Source: CAD feature listing. Evaluate the final solid. Frame: model axes, mm. A direction names the side the tool comes from. Give positions to 0.01 mm unless a question says otherwise; leave off trailing zeros. Write each loop counter-clockwise with the first axis right and the second up, starting at its lowest first coordinate (ties: lowest second). Pieces come first, ordered by that corner, then holes. Notation, with made-up numbers: (53.25, -4) -> (83.25, -4) arc R32 ccw to (83.25, 24) -> close; hole circle Ø8 at (-35, 6). An arc over 180 degrees is marked (long way). Answer as a JSON object with one key per item and string values. Group by question number.
Item 1: Section query A-A on z = -35. Return the cut outline in (x, y), plus the area to 3 significant figures.
Item 2: First-contact query: pin 1 Ø7.5 at (x, y) = (35, 4) entering from -Z; pin 2 Ø9 at (x, y) = (20.5, 14) entering from -Z; pin 3 Ø3 at (x, z) = (9, -17.5) entering from +Y. Flat tips, straight axial feed; report the tip coordinate or a pass-through.
Item 3: Section query C-C on y = 23. Return the cut outline in (x, z).
Item 4: Ray query, probe 1 along X at (y, z) = (16.25, -20.5); probe 2 along Z at (x, y) = (19.5, 9.5); probe 3 along Y at (x, z) = (2.25, -35). Return the intervals inside material, ascending. Write a range as from..to.
Item 5: Pull-direction query (X, two-part tool) for faces 4 (the face through (21.2, 3.2, -24.7)), 5 (the face through (37, 4, -31)), 6 (the face through (8.02, 7.15, -35.93)); classes: pulls with the +X half, pulls with the -X half, needs draft (parallel to the pull), parting line crosses it, or undercut.
Item 6: Access query for faces 1 (the face through (21, 0, -2)), 2 (the face through (4.727, 7.082, -2.465)), 3 (the face through (21, 10, -15)). Directions: +Z, -Z, +X, -X, +Y, -Y. A direction counts if a zero-diameter tool reaches every point of the face in a straight line with its end or side. Return the directions, or none.
Item 7: Section query D-D on z = -9. Return the cut outline in (x, y), plus the area to 3 significant figures.
Item 8: Section query B-B on x = 33.5. Return the cut outline in (y, z).
Autodesk Inventor part; units mm, degrees
ref_plane "YZ Plane" through (0, 0, 0) normal (1, 0, 0) x (0, 1, 0)
ref_plane "XZ Plane" through (0, 0, 0) normal (0, 1, 0) x (-1, 0, 0)
ref_plane "XY Plane" through (0, 0, 0) normal (0, 0, 1) x (1, 0, 0)
sketch "Sketch1" plane through (0, 0, 0) normal (1, 0, 0) x (0, 1, 0)
  line L0 (0, 0) -> (0, -5)
  line L1 (0, -5) -> (20, -5)
  line L2 (20, -5) -> (20, -15)
  line L3 (20, -15) -> (0, -15)
  line L4 (0, -15) -> (0, -39.4721)
  line L5 (25, 0) -> (25, -24)
  line L6 (25, -24) -> (7, -24)
  line L7 (7, -24) -> (7, -29.8038)
  line L8 (25, 0) -> (0, 0)
  circle A0 centre (4, -35) radius 3
  arc A1 (0, -39.4721) -> (7, -29.8038) centre (4, -35) ccw
  dimension "d0" = 5
  dimension "d1" = 20
  dimension "d2" = 10
  dimension "d5" = 5
  dimension "d6" = 7
  dimension "d7" = 6
  dimension "d8" = 20
  dimension "d9" = 4
  dimension "d10" = 6
  dimension "d45" = 9
extrude "Extrusion1" add sketch "Sketch1" along normal blind 42
fillet "Fillet1" radius 5 1 edges at (21, 25, 0)
sketch "Sketch2" plane through (0, 7, -24) normal (0, 1, 0) x (1, 0, 0)
  arc A0 (10.8664, 7) -> (31.1336, 7) centre (21, 12) ccw
  line L0 (0, 0) -> (42, 0)
  line L1 (10.8664, 7) -> (3.3664, 19.9904)
  line L2 (10.8664, 7) -> (25.8664, 7) construction
  line L3 (31.1336, 7) -> (38.6336, 19.9904)
  line L4 (31.1336, 7) -> (46.1336, 7) construction
  line L5 (38.6336, 19.9904) -> (3.3664, 19.9904)
  line L6 (0, 0) -> (42, 0)
  point P0 (0, -24)
  point P1 (21, 0)
  dimension "d14" = 11.3
  dimension "d15" = 12
  dimension "d16" = 7
  dimension "d17" = 15
  dimension "d18" = 120
  dimension "d19" = 15
  dimension "d20" = 60
extrude "Extrusion2" cut sketch "Sketch2" along normal through all both and the other way through all
sketch "Sketch3" plane through (42, 0, 0) normal (1, 0, 0) x (0, 0, -1)
  line L0 (29, 7) -> (31, 7)
  line L1 (31, 7) -> (31, 0)
  line L2 (31, 0) -> (43, 0)
  line L3 (43, 0) -> (43, 12)
  line L4 (43, 12) -> (29, 12)
  line L5 (29, 12) -> (29, 7)
  line L6 (15, 20) -> (15, 0)
  point P0 (0, 0)
  dimension "d23" = 7
  dimension "d24" = 16
  dimension "d25" = 2
  dimension "d26" = 12
  dimension "d27" = 14
extrude "Extrusion3" cut sketch "Sketch3" against normal up to surface
sketch "Sketch4" plane through (0, 25, -24) normal (0, 1, 0) x (1, 0, 0)
  circle A0 centre (5.5, -3.5) radius 1.6
  circle A1 centre (36.5, -3.5) radius 1.6
  line L0 (0, 0) -> (0, -19)
  line L1 (42, 0) -> (42, -19)
  line L2 (0, 0) -> (42, 0)
  point P0 (0, -24)
  dimension "d30" = 3.2
  dimension "d31" = 5.5
  dimension "d32" = 5.5
  dimension "d33" = 3.5
  dimension "d34" = 3.5
extrude "Extrusion4" cut sketch "Sketch4" against normal through all
sketch "Sketch5" plane through (0, 0, 0) normal (0, 0, 1) x (1, 0, 0)
  circle A0 centre (5, 5) radius 2.1
  circle A1 centre (37, 5) radius 2.1
  line L0 (0, 0) -> (42, 0)
  line L1 (0, 20) -> (0, 0)
  line L2 (42, 20) -> (42, 0)
  dimension "d37" = 4.2
  dimension "d38" = 5
  dimension "d39" = 5
  dimension "d40" = 5
extrude "Extrusion5" cut sketch "Sketch5" against normal up to next
sketch "Sketch6" plane through (0, 25, -24) normal (0, 1, 0) x (1, 0, 0)
  spline S0 degree 2 poles (24.4322, -4.6341) (24.4322, -4.7612) (24.4049, -5.0608) knots 0 0 0 1 1 1
  spline S1 degree 2 poles (24.4049, -5.0608) (24.3777, -5.3696) (24.3777, -5.5149) knots 0 0 0 1 1 1
  spline S2 degree 2 poles (24.3777, -5.5149) (24.3777, -6.9405) (24.8045, -8.2754) knots 0 0 0 1 1 1
  spline S3 degree 2 poles (24.8045, -8.2754) (24.977, -8.8293) (24.977, -9.0654) knots 0 0 0 1 1 1
  spline S4 degree 2 poles (24.977, -9.0654) (24.977, -9.3832) (24.4776, -9.7374) (24.2506, -9.7374) knots 0 0 0 1 2 2 2
  spline S5 degree 2 poles (24.2506, -9.7374) (24.1507, -9.7374) (23.7693, -9.6465) knots 0 0 0 1 1 1
  spline S6 degree 2 poles (23.7693, -9.6465) (23.288, -9.5285) (22.6796, -9.4559) knots 0 0 0 1 1 1
  line L0 (22.6796, -9.4559) -> (18.3573, -8.9837)
  spline S7 degree 2 poles (18.3573, -8.9837) (17.7398, -8.9292) (17.3766, -8.8384) (17.086, -8.4752) (17.086, -8.1573) knots 0 0 0 1 2 3 3 3
  spline S8 degree 2 poles (17.086, -8.1573) (17.086, -7.9122) (17.4583, -7.5308) (17.6762, -7.5308) knots 0 0 0 1 2 2 2
  spline S9 degree 2 poles (17.6762, -7.5308) (17.876, -7.5308) (18.3845, -7.6307) knots 0 0 0 1 1 1
  spline S10 degree 2 poles (18.3845, -7.6307) (19.12, -7.7669) (23.2608, -8.2572) (23.3879, -8.2572) knots 0 0 0 1 2 2 2
  spline S11 degree 2 poles (23.3879, -8.2572) (23.5332, -8.2572) (23.5332, -8.2027) knots 0 0 0 1 1 1
  spline S12 degree 2 poles (23.5332, -8.2027) (23.5332, -8.003) (23.397, -7.1131) knots 0 0 0 1 1 1
  spline S13 degree 2 poles (23.397, -7.1131) (23.3243, -6.6954) (23.3062, -6.2686) knots 0 0 0 1 1 1
  spline S14 degree 2 poles (23.3062, -6.2686) (23.2517, -5.0518) (23.1246, -4.5614) knots 0 0 0 1 1 1
  spline S15 degree 2 poles (23.1246, -4.5614) (23.0882, -4.407) (23.0882, -4.3344) knots 0 0 0 1 1 1
  spline S16 degree 2 poles (23.0882, -4.3344) (23.0882, -4.0438) (23.4333, -3.7169) (23.6694, -3.7169) knots 0 0 0 1 2 2 2
  spline S17 degree 2 poles (23.6694, -3.7169) (24.0145, -3.7169) (24.4322, -4.2799) (24.4322, -4.6341) knots 0 0 0 1 2 2 2
  point P0 (0, -24)
  point P1 (17.086, -10.4002)
extrude "Extrusion6" add sketch "Sketch6" along normal blind 0.6
equation "\"d32\" = d31"
equation "\"d40\" = d39"
properties material "ABS Plastic"
Worked answers:
{
 "1": {"outline": "(0, 0) -> (8.56, 0) -> (8.56, 1) -> (0, 1) -> close; (0, 7) -> (8.56, 7) -> (8.56, 10) -> (0, 10) -> close", "area": "34.2 mm^2"},
 "2": {"pin 1": "z = -31", "pin 2": "z = -24", "pin 3": "y = 25"},
 "3": {"outline": "(0, -24) -> (42, -24) -> (42, -1) -> (0, -1) -> close; hole circle Ø3.2 at (5.5, -20.5); hole circle Ø3.2 at (36.5, -20.5)"},
 "4": {"probe 1": "0..3.9, 7.1..34.9, 38.1..42", "probe 2": "-24..-15, -5..0", "probe 3": "0..1, 7..10"},
 "5": {"face 4": "undercut", "face 5": "needs draft", "face 6": "pulls with the +X half"},
 "6": {"face 1": "+Z, -Z, +X, -X, -Y", "face 2": "+Z", "face 3": "+X, -X, -Y"},
 "7": {"outline": "(0, 20) -> (42, 20) -> (42, 25) -> (0, 25) -> close", "area": "210 mm^2"},
 "8": {"outline": "(0, -31) -> (7, -31) -> (7, -24) -> (25, -24) -> (25, -5) arc R5 ccw to (20, 0) -> (0, 0) -> (0, -5) -> (20, -5) -> (20, -15) -> (0, -15) -> close"}
}
